Check sheet for the drawn part. Datum: minimum x, y, z corner. Units: mm. A direction names the side the tool comes from. Coordinates: 2 decimals unless noted, no trailing zeros. Order: outer loops, then holes, each group sorted by start corner. A loop starts at its lowest first (then second) coordinate and runs counter-clockwise, first axis right, second up. Notation, with made-up numbers: M 9.5,-7 L 21.5,-7 A27 ccw 21.5,22 Z; hole C 40.25,59.25 d10. An arc over 180 degrees is marked long. Return JSON: item names as keys, results as strings. Group by question number.
Q1. Section check A-A, the plane y = 6. Enter the section's corners in (x, z), then the cut area to 3 significant figures.
Q2. Thickness scan on probe 1 along X at (y, z) = (1.25, 3); probe 2 along X at (y, z) = (11, 10.5); probe 3 along Y at (x, z) = (9.85, 5.5). Record the ranges inside material, lowest first.
Q3. Mould release check, pull along Z, two halves, no side actions. Record for the marked faces 1, 2, 3 and 4: pulls with the +Z half, pulls with the -Z half, needs draft (parallel to the pull), parting line crosses it, or undercut.
Q4. Section check B-B, the plane z = 8.5. Enter the section's corners in (x, y).
Q5. Section check C-C, the plane x = 3. Enter the section's corners in (y, z), then the cut area to 3 significant figures.
Q6. Section check D-D, the plane y = 8. Enter the section's corners in (x, z), then the cut area to 3 significant figures.
Q7. Go/stop test with flat-tipped pins: pin 1 Ø5 at (y, z) = (11, 6.5) entering from +X; pin 2 Ø1.5 at (x, y) = (11.5, 5.5) entering from +Z; pin 3 Ø1.5 at (y, z) = (11, 1.5) entering from -X; pin 4 Ø3 at (x, z) = (13, 1.5) entering from -Y. Record where each tip stops, or that it passes through.
Q8. Access from +Z, -Z, +X, -X, +Y, -Y to the whole of each face (thin tool, end or side, straight path). Record for the marked faces 5, 6 and 7.
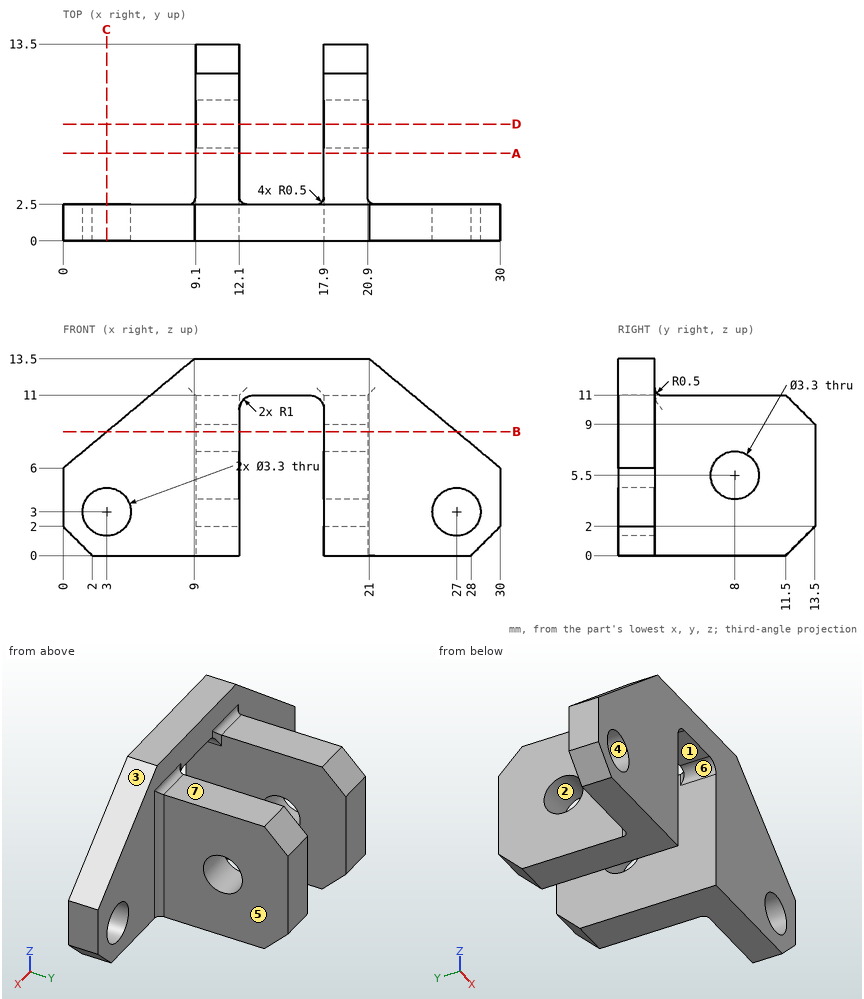
Numbers:
{
 "1": {"outline": "M 9.1,0 L 12.1,0 L 12.1,11 L 9.1,11 Z; M 17.9,0 L 20.9,0 L 20.9,11 L 17.9,11 Z", "area": "66.0 mm2"},
 "2": {"probe 1": "x = 0 to 1.35, 4.65 to 12.1, 17.9 to 25.35, 28.65 to 30", "probe 2": "x = 9.1 to 12.1, 17.9 to 20.9", "probe 3": "y = 0 to 6.35, 9.65 to 13.5"},
 "3": {"face 1": "pulls with the -Z half", "face 2": "undercut", "face 3": "pulls with the +Z half", "face 4": "undercut"},
 "4": {"outline": "M 3,0 L 12.1,0 L 12.1,13.5 L 9.1,13.5 L 9.1,3 A0.5 cw 8.6,2.5 L 3,2.5 Z; M 17.9,0 L 27,0 L 27,2.5 L 21.4,2.5 A0.5 cw 20.9,3 L 20.9,13.5 L 17.9,13.5 Z"},
 "5": {"outline": "M 0,0 L 2.5,0 L 2.5,1.35 L 0,1.35 Z; M 0,4.65 L 2.5,4.65 L 2.5,8.5 L 0,8.5 Z", "area": "13.0 mm2"},
 "6": {"outline": "M 9.1,0 L 12.1,0 L 12.1,3.85 L 9.1,3.85 Z; M 9.1,7.15 L 12.1,7.15 L 12.1,11 L 9.1,11 Z; M 17.9,0 L 20.9,0 L 20.9,3.85 L 17.9,3.85 Z; M 17.9,7.15 L 20.9,7.15 L 20.9,11 L 17.9,11 Z", "area": "46.2 mm2"},
 "7": {"pin 1": "stops at x = 20.9", "pin 2": "stops at z = 11", "pin 3": "stops at x = 9.1", "pin 4": "stops at y = 0"},
 "8": {"face 5": "+Z, -Z, +X, +Y", "face 6": "-Z, +Y, -Y", "face 7": "+Z, +X, -X, +Y"}
}
